Geometry check sheet. Reference: the model listing, model coordinates, mm. A direction names the side the tool comes from. Give positions to 0.01 mm unless a question says otherwise; leave off trailing zeros. Loops run counter-clockwise (first coordinate to the right, second up) from the corner with the lowest first, then second, coordinate; pieces in that order, holes last. Notation, with made-up numbers: (41.5, -8.75) -> (100.5, -8.75) arc R33 ccw to (100.5, 24.25) -> close; hole circle Ø2 at (-23, -33.5). An arc over 180 degrees is marked (long way). One line per item, written item: value. Start each with the question number.
(1) Sectioned sample at D-D, the plane x = 37.5. Record the cut outline in (y, z), then the cut area to 3 significant figures.
(2) Scan lines: line 1 along Y through (x, z) = (48.5, 2); line 2 along X through (y, z) = (14, 0.5); line 3 along X through (y, z) = (72.5, 1.75). Record each from-to range of solid material in increasing order. Write a range as from..to.
(3) Sectioned sample at C-C, the plane x = 0. Record the cut outline in (y, z).
(4) Tool access check on faces 1 (the face through (-6.1, -40, 4)), 2 (the face through (43.53, 95, 4)), 3 (the face through (48, 83.351, 4)). Record the directions out of +Z, -Z, +X, -X, +Y, -Y that give a thin tool (end or side, any length) a straight path to the whole face; none if there is none.
(5) Gauge pin test, flat ends, axial feed: pin 1 Ø10 at (x, y) = (-4, 67) entering from -Z; pin 2 Ø4 at (x, z) = (-4.5, 7) entering from -Y; pin 3 Ø4 at (y, z) = (104, 2.5) entering from -X; pin 4 Ø10 at (x, y) = (21, -38) entering from -Z. Record the tip position at first contact, or that the pin passes through.
(6) Sectioned sample at B-B, the plane z = 6.5. Record the cut outline in (x, y), then the cut area to 3 significant figures.
(7) Sectioned sample at A-A, the plane y = 21. Record the cut outline in (x, z).
(8) Draft check along X on faces 4 (the face through (48, 99.351, 4)), 5 (the face through (-37.743, 14.747, 4.056)), 6 (the face through (51.53, 87, 4)). Enter one of: pulls with the +X half, pulls with the -X half, needs draft (parallel to the pull), parting line crosses it, or undercut.
from build123d import *

# Parameters (mm, degrees)
PAD_DEPTH          = 8
SKETCH001_W        = 12.2
SKETCH001_H        = 8.6
POCKET_DEPTH       = 433.263242
POLARPATTERN_COUNT = 3


with BuildPart() as part:
    # Sketch → Pad (new body)
    with BuildSketch(Plane.XY):
        with BuildLine():
            Line((51.5303, 115.351058), (57.5303, 115.351058))
            Line((57.5303, 115.351058), (57.5303, 17.037153))
            ThreePointArc((-15.362291, 58), (-29.394284, -52.306558), (57.5303, 17.037153))
            Line((43.5303, 67.351058), (-15.362291, 58))
            Line((51.5303, 67.351058), (43.5303, 67.351058))
            Line((51.5303, 75.351058), (51.5303, 67.351058))
            Line((43.5303, 75.351058), (51.5303, 75.351058))
            Line((43.5303, 83.351058), (43.5303, 75.351058))
            Line((51.5303, 83.351058), (43.5303, 83.351058))
            Line((51.5303, 91.351058), (51.5303, 83.351058))
            Line((43.5303, 91.351058), (51.5303, 91.351058))
            Line((43.5303, 99.351058), (43.5303, 91.351058))
            Line((51.5303, 99.351058), (43.5303, 99.351058))
            Line((51.5303, 107.351058), (51.5303, 99.351058))
            Line((43.5303, 107.351058), (51.5303, 107.351058))
            Line((43.5303, 115.351058), (43.5303, 107.351058))
            Line((51.5303, 115.351058), (43.5303, 115.351058))
        make_face()
    extrude(amount=PAD_DEPTH)

    # Sketch001 → Pocket (cut, through all)
    with BuildSketch(Plane.XY.offset(8)):
        with Locations((0, -40)):
            Rectangle(SKETCH001_W, SKETCH001_H)
    pocket = extrude(amount=-POCKET_DEPTH, mode=Mode.SUBTRACT)

    # PolarPattern: Pocket ×3 about axis
    polarpattern_axis = Axis((0, 0, 8), (0, 0, 1))
    for i in range(1, POLARPATTERN_COUNT):
        add(pocket.rotate(polarpattern_axis, i * 360 / POLARPATTERN_COUNT), mode=Mode.SUBTRACT)


solid = part.part
Calculated:
1. outline: (-46.84, 0) -> (14.61, 0) -> (14.61, 8) -> (-46.84, 8) -> close; (23.65, 0) -> (66.39, 0) -> (66.39, 8) -> (23.65, 8) -> close
1. area: 834 mm2
2. line 1: y = -35.32..67.35, 75.35..83.35, 91.35..99.35, 107.35..115.35
2. line 2: x = -58.34..-36.45, -33.14..33.14, 36.45..58.34
2. line 3: x = 51.53..57.53
3. outline: (-60, 0) -> (-44.3, 0) -> (-44.3, 8) -> (-60, 8) -> close; (-35.7, 0) -> (60.44, 0) -> (60.44, 8) -> (-35.7, 8) -> close
4. face 1: +Z, -Z
4. face 2: +Z, -Z, -X, +Y
4. face 3: +Z, -Z, -X
5. pin 1: passes through
5. pin 2: stops at y = -59.95
5. pin 3: stops at x = 51.53
5. pin 4: stops at z = 0
6. outline: (-15.36, 58) arc R60 ccw (long way) to (57.53, 17.04) -> (57.53, 115.35) -> (43.53, 115.35) -> (43.53, 107.35) -> (51.53, 107.35) -> (51.53, 99.35) -> (43.53, 99.35) -> (43.53, 91.35) -> (51.53, 91.35) -> (51.53, 83.35) -> (43.53, 83.35) -> (43.53, 75.35) -> (51.53, 75.35) -> (51.53, 67.35) -> (43.53, 67.35) -> close; hole (-41.41, 16.87) -> (-33.97, 12.57) -> (-27.87, 23.13) -> (-35.31, 27.43) -> close; hole (-6.1, -44.3) -> (6.1, -44.3) -> (6.1, -35.7) -> (-6.1, -35.7) -> close; hole (27.87, 23.13) -> (33.97, 12.57) -> (41.41, 16.87) -> (35.31, 27.43) -> close
6. area: 12,400 mm2
7. outline: (-56.2, 0) -> (-39.03, 0) -> (-39.03, 8) -> (-56.2, 8) -> close; (-29.1, 0) -> (29.1, 0) -> (29.1, 8) -> (-29.1, 8) -> close; (39.03, 0) -> (57.53, 0) -> (57.53, 8) -> (39.03, 8) -> close
8. face 4: needs draft
8. face 5: undercut
8. face 6: pulls with the -X half
